The drawing under review shows one solid part. Ordinate dimensions are in mm from its lowest x, y, z. A direction names the side the tool comes from. Coordinates: 2 decimals unless noted, no trailing zeros. Loops run counter-clockwise (first coordinate to the right, second up) from the corner with the lowest first, then second, coordinate; pieces in that order, holes last. Notation, with made-up numbers: (26.5, 69.25) -> (83.5, 69.25) arc R26 cw to (83.5, 88.25) -> close; hole circle Ø5 at (-20.75, 53). An arc over 180 degrees is marked (long way). Use a Markdown table: item, result.
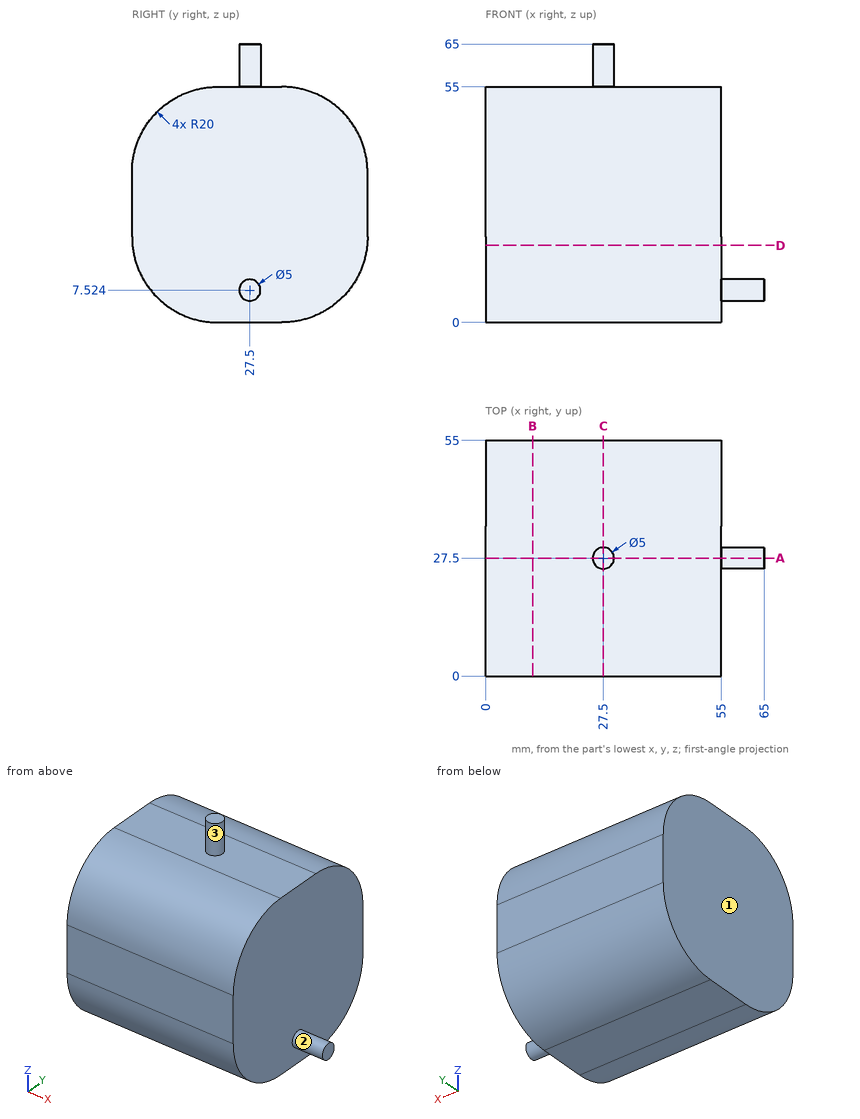
(1) Take a section at D-D on z = 18. Write out the cut boundary in (x, y).
Found:
| item | result |
|---|---|
| outline | (0, 0.1) -> (55, 0.1) -> (55, 54.9) -> (0, 54.9) -> close |
(2) For the marked faces 1, 2 and 3, list the 3-axis set-ups (+Z, -Z, +X, -X, +Y, -Y) from which the entire face can be reached by the end or side of a thin tool; tool diameter is ignored.
Found:
| item | result |
|---|---|
| face 1 | +Z, -Z, -X, +Y, -Y |
| face 2 | +X |
| face 3 | +Z |
(3) Take a section at C-C on x = 27.5. Write out the cut boundary in (y, z).
Found:
| item | result |
|---|---|
| outline | (0, 20) arc R20 ccw to (20, 0) -> (35, 0) arc R20 ccw to (55, 20) -> (55, 35) arc R20 ccw to (35, 55) -> (30, 55) -> (30, 65) -> (25, 65) -> (25, 55) -> (20, 55) arc R20 ccw to (0, 35) -> close |
(4) For line 1 along X through (y, z) = (35, 52.5); line 2 along Z through (x, y) = (42.5, 3.5) (1 decimal), list the stretches that pass through material, from the lowest coordinate up.
Found:
| item | result |
|---|---|
| line 1 | x = 0 to 55 |
| line 2 | z = 8.7 to 46.3 |
(5) For pin 1 Ø2 at (y, z) = (27.5, 57.5) entering from +X; pin 2 Ø12 at (y, z) = (47, 30.5) entering from -X; pin 3 Ø10 at (x, y) = (34, 7) entering from -Z; pin 4 Ø6 at (x, y) = (52, 36.5) entering from +Z, all flat-tipped, find the tip position at first contact; note any pin that passes through.
Found:
| item | result |
|---|---|
| pin 1 | stops at x = 30 |
| pin 2 | stops at x = 0 |
| pin 3 | stops at z = 1.67 |
| pin 4 | stops at z = 55 |
(6) Take a section at B-B on x = 11. Write out the cut boundary in (y, z), plus the area to 3 significant figures.
Found:
| item | result |
|---|---|
| outline | (0, 20) arc R20 ccw to (20, 0) -> (35, 0) arc R20 ccw to (55, 20) -> (55, 35) arc R20 ccw to (35, 55) -> (20, 55) arc R20 ccw to (0, 35) -> close |
| area | 2,680 mm^2 |
(7) Take a section at A-A on y = 27.5. Write out the cut boundary in (x, z), plus the area to 4 significant figures.
Found:
| item | result |
|---|---|
| outline | (0, 0) -> (55, 0) -> (55, 5.02) -> (65, 5.02) -> (65, 10.02) -> (55, 10.02) -> (55, 55) -> (30, 55) -> (30, 65) -> (25, 65) -> (25, 55) -> (0, 55) -> close |
| area | 3,125 mm^2 |
